Part model, mm, in its own coordinate system. Coordinates: 2 decimals unless noted, no trailing zeros. Write each loop counter-clockwise with the first axis right and the second up, starting at its lowest first coordinate (ties: lowest second). Pieces come first, ordered by that corner, then holes. Notation, with made-up numbers: (15.5, 59.25) -> (58.5, 59.25) arc R19 cw to (58.5, 85.25) -> close; hole circle Ø2 at (71.5, 61). An arc over 180 degrees is marked (long way). Write item = value, one per line. Start each with the question number.
Q1. Band-saw the part on C-C, the plane x = -2.85. Give the number of separate pieces and of enclosed holes in the cut face, plus the area to 3 significant figures.
Q2. Band-saw the part on A-A, the plane z = -133.1. List the corners of the cut face in (x, y).
Q3. Band-saw the part on B-B, the plane y = -5. List the corners of the cut face in (x, z), plus the area to 3 significant figures.
Q4. Pin check, flat tips, straight feed: P1, Ø8, axis at y = -5, z = -133.1, coming from the -X side; P2, Ø17.5, axis at y = -28.55, z = -28.55, coming from the -X side. Stop position of each tip, or through.
Q5. Probe line 1 (Y direction, x = -1.6, z = -108); line 2 (Z direction, x = -0.95, y = -5); line 3 (Z direction, x = -4.15, y = -33). List the from-to ranges inside material, lowest first.
Q6. Band-saw the part on D-D, the plane z = -26. List the corners of the cut face in (x, y).
from build123d import *

# Parameters (mm, degrees)
SKETCH1_W           = 138.1
SKETCH1_H           = 57.1
SKETCH1_R           = 2.5
SKETCH1_R_2         = 11
BOSS_EXTRUDE1_DEPTH = 4.7625


with BuildPart() as part:
    # Sketch1 → Boss-Extrude1 (new body)
    with BuildSketch(Plane.ZY):
        with Locations((-69.05, -28.55)):
            Rectangle(SKETCH1_W, SKETCH1_H)
        with Locations(Location((-133.1, -5, 0), (0, 0, 180))):
            Circle(SKETCH1_R, mode=Mode.SUBTRACT)
        with Locations(Location((-133.1, -52.1, 0), (0, 0, 180))):
            Circle(SKETCH1_R, mode=Mode.SUBTRACT)
        with Locations(Location((-28.55, -28.55, 0), (0, 0, 180))):
            Circle(SKETCH1_R_2, mode=Mode.SUBTRACT)
        with Locations(Location((-5, -5, 0), (0, 0, 180))):
            Circle(SKETCH1_R, mode=Mode.SUBTRACT)
        with Locations(Location((-5, -52.1, 0), (0, 0, 180))):
            Circle(SKETCH1_R, mode=Mode.SUBTRACT)
        with BuildLine():
            Line((-108.1, -7.5), (-118.1, -7.5))
            ThreePointArc((-118.1, -7.5), (-120.6, -5), (-118.1, -2.5))
            Line((-118.1, -2.5), (-108.1, -2.5))
            ThreePointArc((-108.1, -2.5), (-105.6, -5), (-108.1, -7.5))
        make_face(mode=Mode.SUBTRACT)
        with BuildLine():
            Line((-108.1, -54.6), (-118.1, -54.6))
            ThreePointArc((-118.1, -54.6), (-120.6, -52.1), (-118.1, -49.6))
            Line((-118.1, -49.6), (-108.1, -49.6))
            ThreePointArc((-108.1, -49.6), (-105.6, -52.1), (-108.1, -54.6))
        make_face(mode=Mode.SUBTRACT)
        with BuildLine():
            Line((-61, -7.5), (-71, -7.5))
            ThreePointArc((-71, -7.5), (-73.5, -5), (-71, -2.5))
            Line((-71, -2.5), (-61, -2.5))
            ThreePointArc((-61, -2.5), (-58.5, -5), (-61, -7.5))
        make_face(mode=Mode.SUBTRACT)
        with BuildLine():
            Line((-61, -54.6), (-71, -54.6))
            ThreePointArc((-71, -54.6), (-73.5, -52.1), (-71, -49.6))
            Line((-71, -49.6), (-61, -49.6))
            ThreePointArc((-61, -49.6), (-58.5, -52.1), (-61, -54.6))
        make_face(mode=Mode.SUBTRACT)
        with BuildLine():
            Line((-84.55, -33.55), (-94.55, -33.55))
            ThreePointArc((-94.55, -33.55), (-99.55, -28.55), (-94.55, -23.55))
            Line((-94.55, -23.55), (-84.55, -23.55))
            ThreePointArc((-84.55, -23.55), (-79.55, -28.55), (-84.55, -33.55))
        make_face(mode=Mode.SUBTRACT)
    extrude(amount=BOSS_EXTRUDE1_DEPTH)


solid = part.part
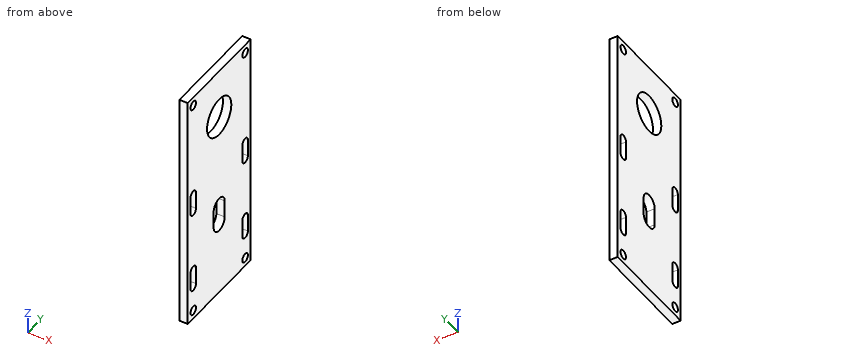
Ans:
q1.separate_pieces = 1
q1.enclosed_holes = 10
q1.area = 6,970 mm2
q2.outline = (-4.76, -57.1) -> (0, -57.1) -> (0, -54.6) -> (-4.76, -54.6) -> close; (-4.76, -49.6) -> (0, -49.6) -> (0, -7.5) -> (-4.76, -7.5) -> close; (-4.76, -2.5) -> (0, -2.5) -> (0, 0) -> (-4.76, 0) -> close
q3.outline = (-4.76, -138.1) -> (0, -138.1) -> (0, -135.6) -> (-4.76, -135.6) -> close; (-4.76, -130.6) -> (0, -130.6) -> (0, -120.6) -> (-4.76, -120.6) -> close; (-4.76, -105.6) -> (0, -105.6) -> (0, -73.5) -> (-4.76, -73.5) -> close; (-4.76, -58.5) -> (0, -58.5) -> (0, -7.5) -> (-4.76, -7.5) -> close; (-4.76, -2.5) -> (0, -2.5) -> (0, 0) -> (-4.76, 0) -> close
q3.area = 467 mm2
q4.P1 = -4.76
q4.P2 = through
q5.line_1 = -57.1 to -54.6, -49.6 to -7.5, -2.5 to 0
q5.line_2 = -138.1 to -135.6, -130.6 to -120.6, -105.6 to -73.5, -58.5 to -7.5, -2.5 to 0
q5.line_3 = -138.1 to -96.83, -82.27 to -38.61, -18.49 to 0
q6.outline = (-4.76, -57.1) -> (0, -57.1) -> (0, -39.25) -> (-4.76, -39.25) -> close; (-4.76, -17.85) -> (0, -17.85) -> (0, 0) -> (-4.76, 0) -> close
